from build123d import *

# Parameters (mm, degrees)
F0_W     = 127
F0_H     = 76.2
F1_DEPTH = 50.8
F2_W     = 101.6
F2_H     = 50.8
F3_DEPTH = 38.1
F4_R     = 7.62


with BuildPart() as f1:
    # F0 (on Front) → F1 (new body)
    with BuildSketch(Plane.XZ):
        Rectangle(F0_W, F0_H)
    extrude(amount=-F1_DEPTH)

    # F2 (on face) → F3 (cut)
    with BuildSketch(Plane.XZ):
        Rectangle(F2_W, F2_H)
    extrude(amount=-F3_DEPTH, mode=Mode.SUBTRACT)

    # F4
    f4_edges = [f1.edges().sort_by_distance(p)[0] for p in [
        (-50.8, 19.05, 25.4),
        (50.8, 19.05, 25.4),
        (50.8, 19.05, -25.4),
        (-50.8, 19.05, -25.4),
        (-63.5, 25.4, -38.1),
        (63.5, 25.4, -38.1),
        (63.5, 25.4, 38.1),
        (-63.5, 25.4, 38.1),
    ]]
    fillet(f4_edges, radius=F4_R)


solid = f1.part
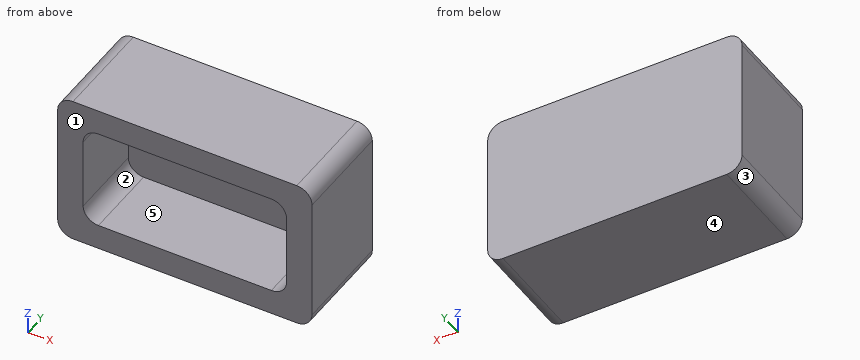
Design review of the part built by this model. Coordinates are the model's own, in mm. Face numbers are marked on the shaded views. A direction names the side the tool comes from. Round coordinates to 2 decimals unless told otherwise and drop trailing zeros. Loops run counter-clockwise (first coordinate to the right, second up) from the corner with the lowest first, then second, coordinate; pieces in that order, holes last. Notation, with made-up numbers: (52, -19) - (68, -19) arc R6 ccw to (68, -12) - close; hole circle Ø8 at (-13.5, -36.75). An arc over 180 degrees is marked (long way). One line per question, with ' | ' between items.
1. We need section A-A, the plane y = 25.5. State the section outline as (x, z) points.
Results are:
outline: (-63.5, -30.48) arc R7.62 ccw to (-55.88, -38.1) - (55.88, -38.1) arc R7.62 ccw to (63.5, -30.48) - (63.5, 30.48) arc R7.62 ccw to (55.88, 38.1) - (-55.88, 38.1) arc R7.62 ccw to (-63.5, 30.48) - close; hole (-50.8, -17.78) arc R7.62 ccw to (-43.18, -25.4) - (43.18, -25.4) arc R7.62 ccw to (50.8, -17.78) - (50.8, 17.78) arc R7.62 ccw to (43.18, 25.4) - (-43.18, 25.4) arc R7.62 ccw to (-50.8, 17.78) - close
2. Clearance check with a flat-ended pin moving along its axis: P1, Ø15, axis at x = 23.5, z = -5, coming from the -Y side. State where the tip first meets the part, or that it passes through.
Results are:
P1: stops at y = 38.1
3. We need section C-C, the plane z = -11. State the section outline as (x, y) points, and give its area (3 significant figures).
Results are:
outline: (-63.5, 0) - (-50.8, 0) - (-50.8, 38.1) - (50.8, 38.1) - (50.8, 0) - (63.5, 0) - (63.5, 50.8) - (-63.5, 50.8) - close | area: 2,580 mm²
4. For the marked faces 4 and 5, list the 3-axis set-ups (+Z, -Z, +X, -X, +Y, -Y) from which the entire face can be reached by the end or side of a thin tool; tool diameter is ignored.
Results are:
face 4: -Z, +X, -X, +Y, -Y | face 5: -Y
5. For L1, parallel to Z at x = -9, y = 10.5; L2, parallel to X at y = 18, z = -6; L3, parallel to Y at x = -12.5, z = 13.5, list the stretches that pass through material, from the lowest coordinate up. Write a range as [from, to].
Results are:
L1: z = [-38.1, -25.4], [25.4, 38.1] | L2: x = [-63.5, -50.8], [50.8, 63.5] | L3: y = [38.1, 50.8]
6. Draft analysis for pull direction Z (two halves, no side actions). For the marked faces 1, 2 and 3, state which applies: released by +Z, released by -Z, zero draft, split by the parting line, or undercut.
Results are:
face 1: zero draft | face 2: undercut | face 3: released by -Z
7. We need section B-B, the plane x = -38. State the section outline as (y, z) points, and give its area (3 significant figures).
Results are:
outline: (0, -38.1) - (50.8, -38.1) - (50.8, 38.1) - (0, 38.1) - (0, 25.4) - (38.1, 25.4) - (38.1, -25.4) - (0, -25.4) - close | area: 1,940 mm²
